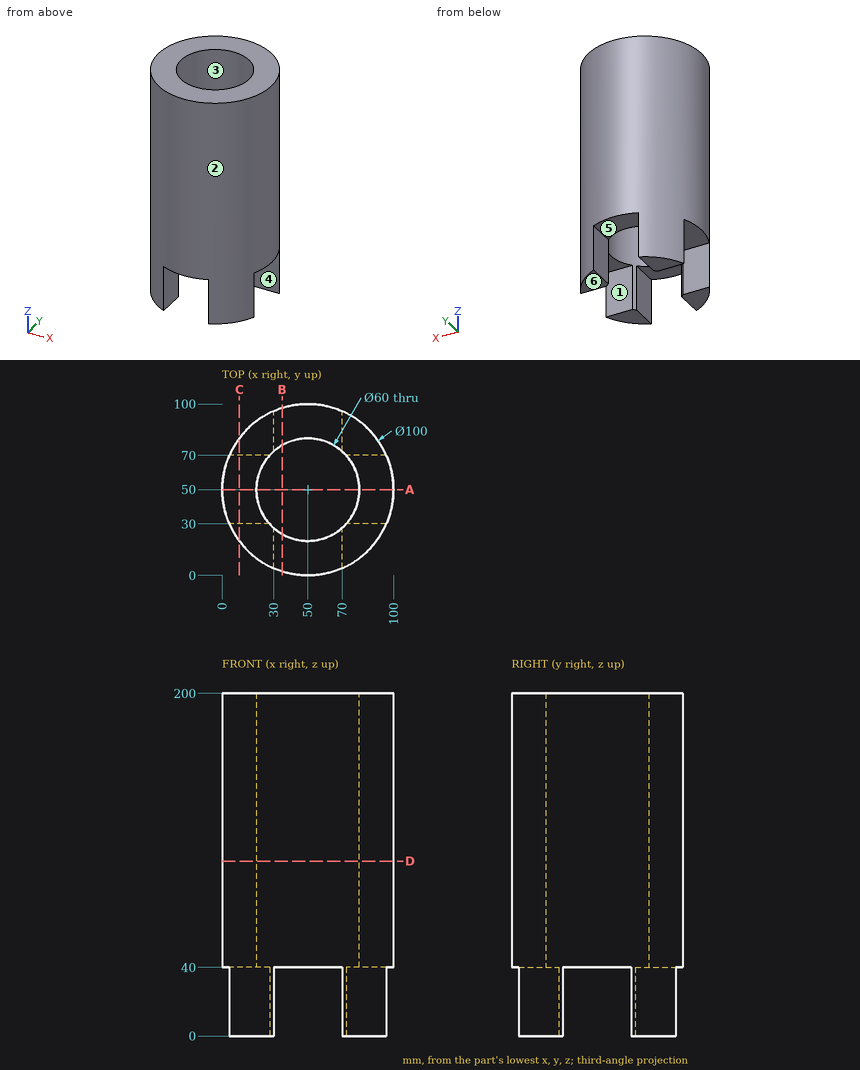
Here's the drawing with two shaded views (mm, measured from the low corner). I have some questions. A direction names the side the tool comes from. Round coordinates to 2 decimals unless told otherwise and drop trailing zeros. Order: outer loops, then holes, each group sorted by start corner. A loop starts at its lowest first (then second) coordinate and runs counter-clockwise, first axis right, second up. Notation, with made-up numbers: (40.5, -4) -> (57.5, -4) arc R26 cw to (57.5, 25) -> close; hole circle Ø11 at (-29, 50.5). An arc over 180 degrees is marked (long way). Use a Markdown table: item, result. Add a question column.
(1) I need wall thicknesses on line 1 along Y through (x, z) = (50, 127.5); line 2 along X through (y, z) = (38, 53.5); line 3 along Y through (x, z) = (22.5, 65). Which ranges of each line are inside material? Lowest first, please.
(2) Suppose I cut it at C-C, the plane x = 10. Please give me the cut outline in (y, z).
(3) Suppose I cut it at D-D, the plane z = 102. Please give me the cut outline in (x, y).
(4) Suppose I cut it at A-A, the plane y = 50. Please give me the cut outline in (x, z).
(5) For pin 1 Ø8.5 at (x, y) = (55, 79.5) entering from -Z; pin 2 Ø7 at (x, z) = (84, 26) entering from +Y; pin 3 Ø19 at (y, z) = (81.5, 16) entering from +X; pin 4 Ø2 at (x, y) = (75, 66) entering from +Z, each with a flat end and sliding along its axis, tell me the tip position at first contact or that it passes through.
(6) Suppose I cut it at B-B, the plane x = 35. Please give me the cut outline in (y, z), and give its area (3 significant figures).
(7) For the marked faces 4, 5 and 6, which set-ups out of +Z, -Z, +X, -X, +Y, -Y let a thin tool reach every point of the face, with its end or its side?
(8) If we mould it in two halves opening along X, with no side actions, what happens to the marked faces 1, 2 and 3? For each: released by +X, released by -X, zero draft, split by the parting line, or undercut.
Verdict:
| question | item | result |
|---|---|---|
| 1 | line 1 | 0 to 20, 80 to 100 |
| 1 | line 2 | 1.46 to 22.5, 77.5 to 98.54 |
| 1 | line 3 | 8.24 to 38.01, 61.99 to 91.76 |
| 2 | outline | (20, 0) -> (30, 0) -> (30, 40) -> (70, 40) -> (70, 0) -> (80, 0) -> (80, 200) -> (20, 200) -> close |
| 3 | outline | circle Ø100 at (50, 50); hole circle Ø60 at (50, 50) |
| 4 | outline | (0, 40) -> (20, 40) -> (20, 200) -> (0, 200) -> close; (80, 40) -> (100, 40) -> (100, 200) -> (80, 200) -> close |
| 5 | pin 1 | z = 40 |
| 5 | pin 2 | y = 89.62 |
| 5 | pin 3 | x = 94.9 |
| 5 | pin 4 | z = 200 |
| 6 | outline | (2.3, 40) -> (24.02, 40) -> (24.02, 200) -> (2.3, 200) -> close; (75.98, 40) -> (97.7, 40) -> (97.7, 200) -> (75.98, 200) -> close |
| 6 | area | 6,950 mm2 |
| 7 | face 4 | -Z, +X, -X |
| 7 | face 5 | -Z, +Y, -Y |
| 7 | face 6 | -Z, +X, -X, +Y, -Y |
| 8 | face 1 | zero draft |
| 8 | face 2 | split by the parting line |
| 8 | face 3 | undercut |
